Can you work these out from the model? Positions are in its coordinate system, mm. A direction names the side the tool comes from. Coordinates: 2 decimals unless noted, no trailing zeros. Loops run counter-clockwise (first coordinate to the right, second up) from the corner with the lowest first, then second, coordinate; pieces in that order, holes last.
```python
from build123d import *

# Parameters (mm, degrees)
F0_R     = 1.5
F1_DEPTH = 1.5
F2_W     = 20
F2_H     = 1
F3_DEPTH = 27
F4_W     = 10
F4_H     = 5
F4_W_2   = 5
F4_H_2   = 20
F5_DEPTH = 10
F6_SIZE  = 2


with BuildPart() as f1:
    # F0 (on Top) → F1 (new body)
    with BuildSketch(Plane.XY):
        with BuildLine():
            ThreePointArc((30, 22.5), (28.535534, 26.035534), (25, 27.5))
            Line((25, 27.5), (-25, 27.5))
            ThreePointArc((-25, 27.5), (-28.535534, 26.035534), (-30, 22.5))
            Line((-30, 22.5), (-30, -22.5))
            ThreePointArc((-30, -22.5), (-28.535534, -26.035534), (-25, -27.5))
            Line((-25, -27.5), (25, -27.5))
            ThreePointArc((25, -27.5), (28.535534, -26.035534), (30, -22.5))
            Line((30, -22.5), (30, 22.5))
        make_face()
        with Locations((-25, -22.5)):
            Circle(F0_R, mode=Mode.SUBTRACT)
        with Locations((25, -22.5)):
            Circle(F0_R, mode=Mode.SUBTRACT)
        with Locations((-25, 22.5)):
            Circle(F0_R, mode=Mode.SUBTRACT)
        with Locations((25, 22.5)):
            Circle(F0_R, mode=Mode.SUBTRACT)
    extrude(amount=-F1_DEPTH)

    # F2 (on face) → F3 (join)
    with BuildSketch(Plane.XY):
        with Locations((-14.875233, 0)):
            Rectangle(F2_W, F2_H)
        with Locations((-14.875233, 4)):
            Rectangle(F2_W, F2_H)
        with Locations((-14.875233, 8)):
            Rectangle(F2_W, F2_H)
        with Locations((-14.875233, -4)):
            Rectangle(F2_W, F2_H)
        with Locations((-14.875233, -8)):
            Rectangle(F2_W, F2_H)
    extrude(amount=F3_DEPTH)

    # F4 (on face) → F5 (join)
    with BuildSketch(Plane.XY):
        with Locations((0, 22.5)):
            Rectangle(F4_W, F4_H)
        with Locations((0, -22.5)):
            Rectangle(F4_W, F4_H)
        with Locations((25, 0)):
            Rectangle(F4_W_2, F4_H_2)
    extrude(amount=F5_DEPTH)

    # F6
    f6_edges = [f1.edges().sort_by_distance(p)[0] for p in [
        (0, 20, 10),
        (22.5, 0, 10),
        (0, -20, 10),
    ]]
    chamfer(f6_edges, length=F6_SIZE)


solid = f1.part
```
(1) I want a section at B-B on x = 7.5. Write out the boundary of the cut face in (y, z).
Check values:
outline: (-27.5, -1.5) - (27.5, -1.5) - (27.5, 0) - (-27.5, 0) - close
(2) If I drill on probe 1 along Y at (x, z) = (-25, -0.4); probe 2 along Y at (x, z) = (-16, 21.5); probe 3 along X at (y, z) = (4, 4), over which ranges is the centre line in solid material (lowest first)?
Check values:
probe 1: y = -27.5 to -24, -21 to 21, 24 to 27.5
probe 2: y = -8.5 to -7.5, -4.5 to -3.5, -0.5 to 0.5, 3.5 to 4.5, 7.5 to 8.5
probe 3: x = -24.88 to -4.88, 22.5 to 27.5
(3) I'm going to push flat-ended pins straight in: pin 1 (16 mm diameter, centred on x = -10, z = 13.5, fed in from +Y); pin 2 (1 mm diameter, centred on y = 7.5, z = 1.5, fed in from +X); pin 3 (3.5 mm diameter, centred on x = -25, y = -22.5, fed in from +Z). Where does each tip first touch, or does it pass through?
Check values:
pin 1: stops at y = 25
pin 2: stops at x = 27.5
pin 3: stops at z = 0
(4) I want a section at A-A on z = 17.75. Write out the boundary of the cut face in (x, y).
Check values:
outline: (-24.88, -8.5) - (-4.88, -8.5) - (-4.88, -7.5) - (-24.88, -7.5) - close; (-24.88, -4.5) - (-4.88, -4.5) - (-4.88, -3.5) - (-24.88, -3.5) - close; (-24.88, -0.5) - (-4.88, -0.5) - (-4.88, 0.5) - (-24.88, 0.5) - close; (-24.88, 3.5) - (-4.88, 3.5) - (-4.88, 4.5) - (-24.88, 4.5) - close; (-24.88, 7.5) - (-4.88, 7.5) - (-4.88, 8.5) - (-24.88, 8.5) - close
(5) Which directions (+Z, -Z, +X, -X, +Y, -Y) give clear straight access to the entire face, cutting with the end or side of a thin tool? Please do faces 1 (the flat face through (-15, -7.5, 13)), 2 (the flat face through (0, 21, 9)), 3 (the flat face through (0, -25, 5)).
Check values:
face 1: +Z, -X
face 2: +Z, +X, -X
face 3: +Z, +X, -X, -Y
(6) If we mould it in two halves opening along X, with no side actions, what happens to faces 4 (the cylindrical face through (23.89, -21.49, -0.74)), 5 (the flat face through (5, -23, 5)), 6 (the flat face through (-15, 0.5, 13))? For each: released by +X, released by -X, zero draft, split by the parting line, or undercut.
Check values:
face 4: undercut
face 5: released by +X
face 6: zero draft
(7) I want a section at C-C on y = -14. Write out the boundary of the cut face in (x, z).
Check values:
outline: (-30, -1.5) - (30, -1.5) - (30, 0) - (-30, 0) - close
